```python
from build123d import *

# Parameters (mm, degrees)
BOSS_EXTRUDE1_DEPTH = 2.5
SKETCH2_W           = 18.3
SKETCH2_H           = 2
BOSS_EXTRUDE2_DEPTH = 14
SKETCH3_W           = 18.3
SKETCH3_H           = 3
BOSS_EXTRUDE3_DEPTH = 22.98
SKETCH4_W           = 5
SKETCH4_H           = 9.60227247
SKETCH4_W_2         = 6.06
SKETCH4_H_2         = 22.98
CUT_EXTRUDE1_DEPTH  = 3
SKETCH5_W           = 6.06
SKETCH5_H           = 14
CUT_EXTRUDE2_DEPTH  = 2


with BuildPart() as part:
    # Sketch1 → Boss-Extrude1 (new body)
    with BuildSketch(Plane(origin=(0, 0, 0), x_dir=(1, 0, 0), z_dir=(0, 1, 0))):
        with BuildLine():
            Line((-9.15, -3.5), (-9.15, 1.930673458))
            Line((-9.15, 1.930673458), (-6.075, 1.930673458))
            ThreePointArc((-6.075, 1.930673458), (-4.825, -2.3), (-3.575, 1.930673458))
            Line((-3.575, 1.930673458), (-0.575, 1.930673458))
            Line((-0.575, 1.930673458), (-0.575, -2.281126238))
            Line((-0.575, -2.281126238), (0.575, -2.281126238))
            Line((0.575, -2.281126238), (0.575, 1.930673458))
            Line((0.575, 1.930673458), (3.575, 1.930673458))
            ThreePointArc((3.575, 1.930673458), (4.825, -2.3), (6.075, 1.930673458))
            Line((6.075, 1.930673458), (9.15, 1.930673458))
            Line((9.15, 1.930673458), (9.15, -3.5))
            Line((9.15, -3.5), (9.15, -5.5))
            Line((9.15, -5.5), (-9.15, -5.5))
            Line((-9.15, -5.5), (-9.15, -3.5))
        make_face()
    extrude(amount=BOSS_EXTRUDE1_DEPTH)

    # Sketch2 → Boss-Extrude2 (add)
    with BuildSketch(Plane(origin=(0, 2.5, 0), x_dir=(1, 0, 0), z_dir=(0, 1, 0))):
        with Locations((0, -4.5)):
            Rectangle(SKETCH2_W, SKETCH2_H)
    extrude(amount=BOSS_EXTRUDE2_DEPTH)

    # Sketch3 → Boss-Extrude3 (add)
    with BuildSketch(Plane(origin=(0, 0, 3.5), x_dir=(-1, 0, 0), z_dir=(0, 0, -1))):
        with Locations((0, 15)):
            Rectangle(SKETCH3_W, SKETCH3_H)
    extrude(amount=BOSS_EXTRUDE3_DEPTH)

    # Sketch4 → Cut-Extrude1 (cut)
    with BuildSketch(Plane(origin=(0, 16.5, 0), x_dir=(1, 0, 0), z_dir=(0, 1, 0))):
        with Locations((1.41, 12.678863765)):
            Rectangle(SKETCH4_W, SKETCH4_H)
        with Locations((-6.12, 7.99)):
            Rectangle(SKETCH4_W_2, SKETCH4_H_2)
    extrude(amount=-CUT_EXTRUDE1_DEPTH, mode=Mode.SUBTRACT)

    # Sketch5 → Cut-Extrude2 (cut)
    with BuildSketch(Plane.XY.offset(5.5)):
        with Locations((-6.12, 9.5)):
            Rectangle(SKETCH5_W, SKETCH5_H)
    extrude(amount=-CUT_EXTRUDE2_DEPTH, mode=Mode.SUBTRACT)


solid = part.part
```
Work out the finished part from the listing and answer in its coordinate system (mm). A direction names the side the tool comes from. Coordinates: 2 decimals unless noted, no trailing zeros. Loops run counter-clockwise (first coordinate to the right, second up) from the corner with the lowest first, then second, coordinate; pieces in that order, holes last. Notation, with made-up numbers: (-33.5, 44) - (11.5, 44) arc R22 cw to (11.5, 83) - close; hole circle Ø11 at (11, 3.5). An arc over 180 degrees is marked (long way). Use a Markdown table: item, result.
Item 1: Find section B-B, the plane z = -8.5. Determine the outline of the cut face in (x, y), and give its area (3 significant figures).
Evaluation:
| item | result |
|---|---|
| outline | (-3.09, 13.5) - (-1.09, 13.5) - (-1.09, 16.5) - (-3.09, 16.5) - close; (3.91, 13.5) - (9.15, 13.5) - (9.15, 16.5) - (3.91, 16.5) - close |
| area | 21.7 mm2 |
Item 2: The mould has two halves that part along Z. Classify faces 1 (the flat face through (3.91, 15, -13)), 2 (the flat face through (3, 15, -19.48)), 3 (the flat face through (3, 16.5, -7)): +Z half, -Z half, draft (parallel to the pull), parting line (faces both ways), or undercut.
Evaluation:
| item | result |
|---|---|
| face 1 | undercut |
| face 2 | -Z half |
| face 3 | draft |
Item 3: Find section D-D, the plane x = 5. Determine the outline of the cut face in (y, z).
Evaluation:
| item | result |
|---|---|
| outline | (0, 2.29) - (2.5, 2.29) - (2.5, 3.5) - (13.5, 3.5) - (13.5, -19.48) - (16.5, -19.48) - (16.5, 5.5) - (0, 5.5) - close |
Item 4: Given pin 1 Ø1.2 at (x, y) = (8.5, 1) entering from -Z; pin 2 Ø2 at (x, z) = (5, -4.5) entering from -Y; pin 3 Ø3 at (x, y) = (1.5, 6.5) entering from -Z, each flat-ended and moving along its own axis, determine where each tip first touches the part or whether it passes through.
Evaluation:
| item | result |
|---|---|
| pin 1 | stops at z = -1.93 |
| pin 2 | stops at y = 13.5 |
| pin 3 | stops at z = 3.5 |
Item 5: Consider probe 1 along X at (y, z) = (1.2, 0) (3 decimals); probe 2 along Z at (x, y) = (1, 12.5); probe 3 along Y at (x, z) = (-0.5, -4). Determine where each line is inside the solid, lowest interval first. Write a range as from..to.
Evaluation:
| item | result |
|---|---|
| probe 1 | x = -9.15..-7.125, -2.525..-0.575, 0.575..2.525, 7.125..9.15 |
| probe 2 | z = 3.5..5.5 |
| probe 3 | y = 13.5..16.5 |
Item 6: Find section A-A, the plane y = 14.25. Determine the outline of the cut face in (x, z).
Evaluation:
| item | result |
|---|---|
| outline | (-3.09, -19.48) - (9.15, -19.48) - (9.15, 5.5) - (-3.09, 5.5) - close; hole (-1.09, -17.48) - (3.91, -17.48) - (3.91, -7.88) - (-1.09, -7.88) - close |
Item 7: For faces 4 (the flat face through (-0.575, 1, 0)), 5 (the cylindrical face through (4.74, 1.23, 2.3)), 6 (the flat face through (4.5, 13.5, -7.8)), 7 (the flat face through (-3.09, 14, -4)), determine the directions among +Z, -Z, +X, -X, +Y, -Y from which every point of the face is accessible in a straight line to the end or side of a thin tool.
Evaluation:
| item | result |
|---|---|
| face 4 | -Z, -Y |
| face 5 | -Y |
| face 6 | -Z, +X, -X |
| face 7 | +Z, -Z, -X, +Y |
Item 8: Find section C-C, the plane z = 0. Determine the outline of the cut face in (x, y) (3 decimals), and give its area (3 significant figures).
Evaluation:
| item | result |
|---|---|
| outline | (-9.15, 0) - (-7.125, 0) - (-7.125, 2.5) - (-9.15, 2.5) - close; (-3.09, 13.5) - (9.15, 13.5) - (9.15, 16.5) - (-3.09, 16.5) - close; (-2.525, 0) - (-0.575, 0) - (-0.575, 2.5) - (-2.525, 2.5) - close; (0.575, 0) - (2.525, 0) - (2.525, 2.5) - (0.575, 2.5) - close; (7.125, 0) - (9.15, 0) - (9.15, 2.5) - (7.125, 2.5) - close |
| area | 56.6 mm2 |
